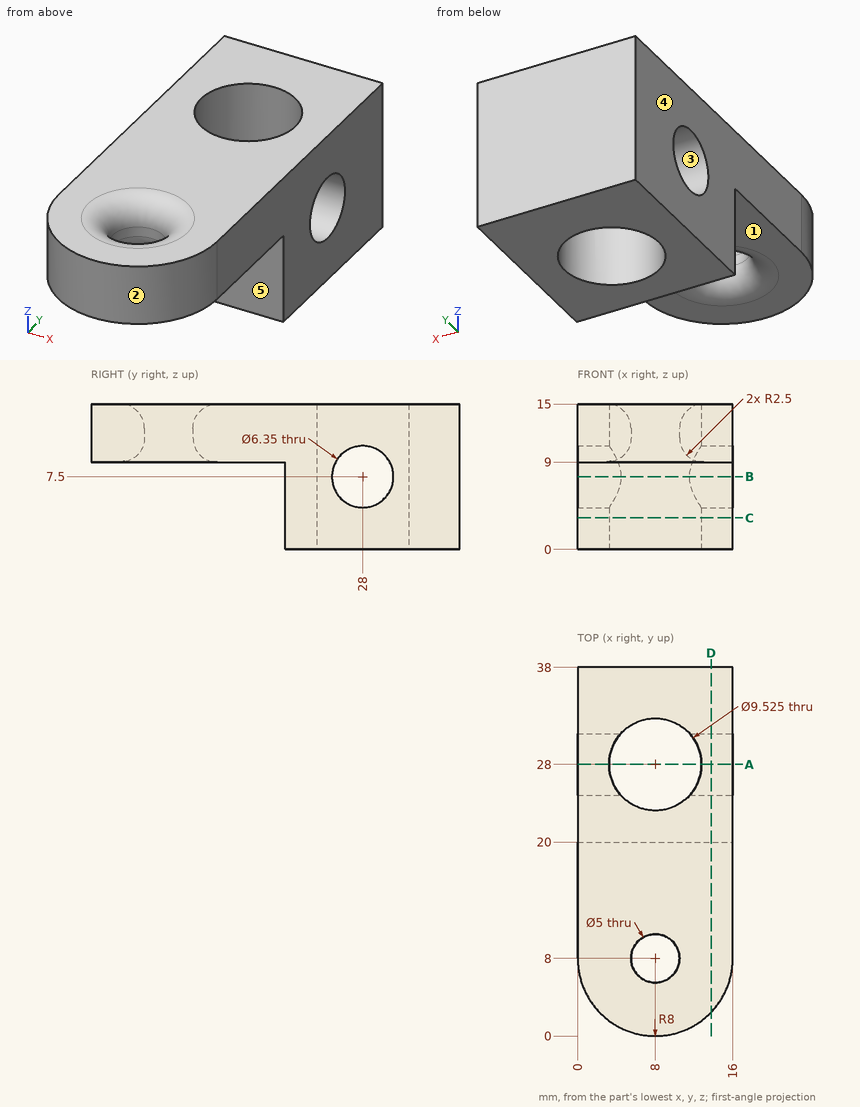
Here's the drawing with two shaded views (mm, measured from the low corner). I have some questions. A direction names the side the tool comes from. Coordinates: 2 decimals unless noted, no trailing zeros. Loops run counter-clockwise (first coordinate to the right, second up) from the corner with the lowest first, then second, coordinate; pieces in that order, holes last. Notation, with made-up numbers: (35, 8.5) -> (67, 8.5) arc R28 cw to (67, 31.5) -> close; hole circle Ø1 at (60, 67.25). An arc over 180 degrees is marked (long way). Put each result on its own line as item: value. Start each with the question number.
Q1. I'm going to push flat-ended pins straight in: P1, Ø7, axis at x = 4.5, z = 3, coming from the -Y side; P2, Ø8, axis at x = 8, y = 8, coming from the -Z side. Where does each tip first touch, or does it pass through?
Q2. Thinking about a two-plate mould opening in Z: for the marked faces 1, 2 and 3, which applies, pulls with the +Z half, pulls with the -Z half, needs draft (parallel to the pull), parting line crosses it, or undercut?
Q3. I want a section at A-A (y = 28). Write out the boundary of the cut face in (x, z) (1 decimal).
Q4. I want a section at B-B (z = 7.5). Write out the boundary of the cut face in (x, y) (1 decimal).
Q5. I want a section at C-C (z = 3.25). Write out the boundary of the cut face in (x, y) (1 decimal).
Q6. If I drill on line 1 (Y direction, x = 8, z = 12.1); line 2 (X direction, y = 8, z = 11.95); line 3 (Y direction, x = 8, z = 3.25), over which ranges is the centre line in solid material (lowest first)? Write a range as [from, to].
Q7. For the marked faces 4 and 5, which set-ups out of +Z, -Z, +X, -X, +Y, -Y let a thin tool reach every point of the face, with its end or its side?
Q8. I want a section at D-D (x = 13.75). Write out the boundary of the cut face in (y, z) (3 decimals).
Taken from the geometry:
1. P1: stops at y = 20
1. P2: stops at z = 9.21
2. face 1: pulls with the -Z half
2. face 2: needs draft
2. face 3: undercut
3. outline: (0, 0) -> (3.2, 0) -> (3.2, 4.3) -> (0, 4.3) -> close; (0, 10.7) -> (3.2, 10.7) -> (3.2, 15) -> (0, 15) -> close; (12.8, 0) -> (16, 0) -> (16, 4.3) -> (12.8, 4.3) -> close; (12.8, 10.7) -> (16, 10.7) -> (16, 15) -> (12.8, 15) -> close
4. outline: (0, 20) -> (16, 20) -> (16, 24.8) -> (11.5, 24.8) arc R4.8 cw to (4.5, 24.8) -> (0, 24.8) -> close; (0, 31.2) -> (4.5, 31.2) arc R4.8 cw to (11.5, 31.2) -> (16, 31.2) -> (16, 38) -> (0, 38) -> close
5. outline: (0, 20) -> (16, 20) -> (16, 38) -> (0, 38) -> close; hole circle Ø9.5 at (8, 28)
6. line 1: y = [0, 5.5], [10.5, 23.24], [32.76, 38]
6. line 2: x = [0, 5.5], [10.5, 16]
6. line 3: y = [20, 23.24], [32.76, 38]
7. face 4: +Z, -Z, -X, +Y, -Y
7. face 5: -Z, +X, -X, -Y
8. outline: (2.438, 9) -> (20, 9) -> (20, 0) -> (38, 0) -> (38, 15) -> (2.438, 15) -> close; hole circle Ø6.35 at (28, 7.5)
